Input: part model. Units: mm. Frame: model coordinates. Face numbers are marked on the shaded views. A direction names the side the tool comes from. Round coordinates to 2 decimals unless told otherwise and drop trailing zeros. Write each loop counter-clockwise with the first axis right and the second up, starting at its lowest first coordinate (ties: lowest second). Pieces come first, ordered by that corner, then holes. Notation, with made-up numbers: (40, 61) - (80, 61) arc R16 ccw to (80, 71) - close; hole circle Ø7 at (52, -4). An arc over 180 degrees is marked (long way). Use one line per item in the form item = value.
```python
from build123d import *

# Parameters (mm, degrees)
SKETCH1_R                                           = 44.45
SKETCH1_R_2                                         = 39.45
BOSS_EXTRUDE1_DEPTH                                 = 20
BOSS_EXTRUDE2_START                                 = 20
SKETCH4_R                                           = 44.45
SKETCH4_R_2                                         = 6
BOSS_EXTRUDE2_DEPTH                                 = 20
SKETCH5_R                                           = 44.45
SKETCH5_R_2                                         = 33.45
CUT_EXTRUDE1_DEPTH                                  = 3
LPATTERN1_COUNT                                     = 4
LPATTERN1_PITCH                                     = 5
CBORE_FOR_4_BINDING_HEAD_MACHINE_SCREW3_D           = 3.2639
CBORE_FOR_4_BINDING_HEAD_MACHINE_SCREW3_CBORE_D     = 6.74624
CBORE_FOR_4_BINDING_HEAD_MACHINE_SCREW3_CBORE_DEPTH = 14.4272
CIRPATTERN2_COUNT                                   = 3


with BuildPart() as part:
    # Sketch1 → Boss-Extrude1 (new body)
    with BuildSketch(Plane.XY):
        Circle(SKETCH1_R)
        Circle(SKETCH1_R_2, mode=Mode.SUBTRACT)
    extrude(amount=BOSS_EXTRUDE1_DEPTH)

    # Sketch4 → Boss-Extrude2 (add)
    with BuildSketch(Plane(origin=(0, 0, 0), x_dir=(-1, 0, 0), z_dir=(0, 0, -1)).offset(BOSS_EXTRUDE2_START)):
        Circle(SKETCH4_R)
        Circle(SKETCH4_R_2, mode=Mode.SUBTRACT)
    extrude(amount=-BOSS_EXTRUDE2_DEPTH)

    # Sketch5 → Cut-Extrude1 (cut)
    with BuildSketch(Plane(origin=(0, 0, -20), x_dir=(-1, 0, 0), z_dir=(0, 0, -1))):
        Circle(SKETCH5_R)
        Circle(SKETCH5_R_2, mode=Mode.SUBTRACT)
    cut_extrude1 = extrude(amount=-CUT_EXTRUDE1_DEPTH, mode=Mode.SUBTRACT)

    # LPattern1: Cut-Extrude1 ×4
    with Locations(*[(0, 0, i * LPATTERN1_PITCH) for i in range(1, LPATTERN1_COUNT)]):
        add(cut_extrude1, mode=Mode.SUBTRACT)

    # CBORE for #4 Binding Head Machine Screw3 (through all)
    with Locations(Plane(origin=(0, 0, -17), x_dir=(-1, 0, 0), z_dir=(0, 0, -1))):
        with Locations((0, 41.95)):
            cbore_for_4_binding_head_machine_screw3 = CounterBoreHole(CBORE_FOR_4_BINDING_HEAD_MACHINE_SCREW3_D / 2, CBORE_FOR_4_BINDING_HEAD_MACHINE_SCREW3_CBORE_D / 2, CBORE_FOR_4_BINDING_HEAD_MACHINE_SCREW3_CBORE_DEPTH)

    # CirPattern2: CBORE for #4 Binding Head Machine Screw3 ×3 about axis
    cirpattern2_axis = Axis((0, 0, 0), (0, 0, 1))
    for i in range(1, CIRPATTERN2_COUNT):
        add(cbore_for_4_binding_head_machine_screw3.rotate(cirpattern2_axis, i * 360 / CIRPATTERN2_COUNT), mode=Mode.SUBTRACT)


solid = part.part
```
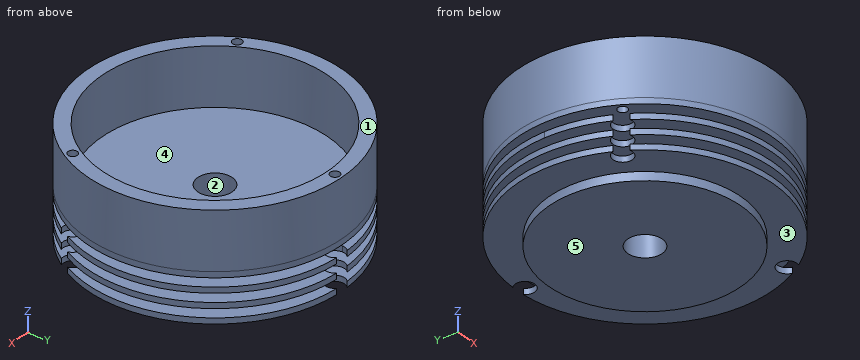
(1) Cut plane A-A on x = 0. Count the separate pieces of the cut face and the enclosed holes in it, then the cut area to 3 significant figures.
Derived:
separate_pieces = 3
enclosed_holes = 0
area = 1,370 mm^2
(2) Access query for the marked faces 3, 4 and 5. Directions: +Z, -Z, +X, -X, +Y, -Y. A direction counts if a zero-diameter tool reaches every point of the face in a straight line with its end or side. Return the directions, or none.
Derived:
face_3 = -Z
face_4 = +Z
face_5 = -Z, +X, -X, +Y, -Y
(3) First-contact query: pin 1 Ø5 at (x, y) = (-36.33, -20.97) entering from -Z; pin 2 Ø14 at (x, y) = (0, 0) entering from +Z; pin 3 Ø12 at (y, z) = (31, 5.5) entering from -X; pin 4 Ø2 at (x, y) = (36.33, -20.98) entering from -Z. Flat tips, straight axial feed; report the tip coordinate or a pass-through.
Derived:
pin_1 = -2
pin_2 = 0
pin_3 = -36.75
pin_4 = through
(4) Cut plane B-B on z = 6.5. Output: boundary loops of the cut face in (x, y) (3 decimals), then the cut area to 3 significant figures.
Derived:
outline = circle Ø88.9 at (0, 0); hole circle Ø78.9 at (0, 0); hole circle Ø3.264 at (-36.33, -20.975); hole circle Ø3.264 at (0, 41.95); hole circle Ø3.264 at (36.33, -20.975)
area = 1,290 mm^2
(5) Draft query along X for the marked faces 1 and 2. Return one class per face: released by +X, released by -X, zero draft, split by the parting line, or undercut.
Derived:
face_1 = zero draft
face_2 = undercut
(6) Material intervals for L1, parallel to Z at x = 39.5, y = -17.5; L2, parallel to Z at x = 22.5, y = -29; L3, parallel to Y at x = 0, z = 6, sorted ascending.
Derived:
L1 = -17 to -15, -12 to -10, -7 to -5, -2 to 20
L2 = -17 to -15, -12 to -10, -7 to -5, -2 to 0
L3 = -44.45 to -39.45, 39.45 to 40.32, 43.58 to 44.45
